For this review, take the finished solid that the model builds, in its own axes (mm). A direction names the side the tool comes from. Coordinates: 2 decimals unless noted, no trailing zeros. Loops run counter-clockwise (first coordinate to the right, second up) from the corner with the lowest first, then second, coordinate; pieces in that order, holes last. Notation, with made-up numbers: (-17, -32.5) -> (-9, -32.5) arc R23 cw to (-9, -16.5) -> close; hole circle Ø3 at (76, -13.75). An arc over 180 degrees is marked (long way). One line per item, written item: value.
from build123d import *

# Parameters (mm, degrees)
SKETCH_W      = 102.2
SKETCH_H      = 83
SKETCH_W_2    = 30
SKETCH_H_2    = 5
SKETCH_W_3    = 2
SKETCH_H_3    = 25
PAD_DEPTH     = 2
SKETCH001_R   = 2.4
SKETCH001_R_2 = 1.2
PAD001_DEPTH  = 6.2
PAD002_DEPTH  = 6.9
PAD003_DEPTH  = 1
SKETCH004_W   = 1.45
SKETCH004_H   = 11.2
PAD004_DEPTH  = 5
SKETCH005_W   = 1.45
SKETCH005_H   = 5
PAD005_DEPTH  = 5
PAD006_DEPTH  = 5
SKETCH007_W   = 107
SKETCH007_H   = 26.1
SKETCH007_W_2 = 102.2
SKETCH007_H_2 = 21.7
PAD007_DEPTH  = 5
SKETCH008_W   = 27
SKETCH008_H   = 2.75
PAD008_DEPTH  = 3.8
CHAMFER_SIZE  = 1
SKETCH009_W   = 46.5
SKETCH009_H   = 26.1
SKETCH009_W_2 = 42.1
SKETCH009_H_2 = 21.7
PAD009_DEPTH  = 5
SKETCH010_W   = 2
SKETCH010_H   = 21.75
PAD010_DEPTH  = 3.8
FILLET_R      = 1.5


with BuildPart() as part:
    # Sketch → Pad (new body)
    with BuildSketch(Plane.XY):
        Rectangle(SKETCH_W, SKETCH_H)
        with Locations((34.1, 17.5)):
            Rectangle(SKETCH_W_2, SKETCH_H_2, mode=Mode.SUBTRACT)
        with Locations((-34.1, 17.5)):
            Rectangle(SKETCH_W_2, SKETCH_H_2, mode=Mode.SUBTRACT)
        with Locations((6, -27)):
            Rectangle(SKETCH_W_3, SKETCH_H_3, mode=Mode.SUBTRACT)
        with Locations((-6, -27)):
            Rectangle(SKETCH_W_3, SKETCH_H_3, mode=Mode.SUBTRACT)
    extrude(amount=PAD_DEPTH)

    # Sketch001 (on Face22 of Pad) → Pad001 (join)
    with BuildSketch(Plane.XY.offset(2)):
        with Locations((-42.5, -25)):
            Circle(SKETCH001_R)
        with Locations((-42.5, -25)):
            Circle(SKETCH001_R_2, mode=Mode.SUBTRACT)
        with Locations((42.5, 25)):
            Circle(SKETCH001_R)
        with Locations((42.5, 25)):
            Circle(SKETCH001_R_2, mode=Mode.SUBTRACT)
    extrude(amount=PAD001_DEPTH)

    # Sketch002 → Pad002 (join)
    with BuildSketch(Plane.XY):
        Polygon((-51.1, 41.5), (51.1, 41.5), (51.1, 5.05), (53.5, 5.05), (53.5, 43.85), (-53.5, 43.85), (-53.5, 5.05), (-51.1, 5.05), align=None)
    pad002 = extrude(amount=PAD002_DEPTH)

    # Mirrored: Pad002 across XZ
    add(pad002.mirror(Plane.XZ))

    # Sketch003 (on Face36 of Mirrored) → Pad003 (join)
    with BuildSketch(Plane.XY.offset(6.9)):
        Polygon((-51.1, 5.05), (-51.1, 41.5), (51.1, 41.5), (51.1, 5.05), (52.05, 5.05), (52.05, 42.45), (-52.05, 42.45), (-52.05, 5.05), align=None)
    pad003 = extrude(amount=PAD003_DEPTH)

    # Mirrored001: Pad003 across XZ
    add(pad003.mirror(Plane.XZ))

    # Sketch004 (on Face3 of Mirrored001) → Pad004 (join)
    with BuildSketch(Plane.XY.offset(2)):
        with Locations((50.375, 0)):
            Rectangle(SKETCH004_W, SKETCH004_H)
    pad004 = extrude(amount=PAD004_DEPTH)

    # Mirrored002: Pad004 across YZ
    add(pad004.mirror(Plane.YZ))

    # Sketch005 (on Face40 of Mirrored002) → Pad005 (join)
    with BuildSketch(Plane.XY.offset(7)):
        with Locations((50.375, 0)):
            Rectangle(SKETCH005_W, SKETCH005_H)
    pad005 = extrude(amount=PAD005_DEPTH)

    # Mirrored003: Pad005 across YZ
    add(pad005.mirror(Plane.YZ))

    # Sketch006 (on Face2 of Mirrored003) → Pad006 (join)
    with BuildSketch(Plane.XZ.offset(2.5)):
        Polygon((49.65, 12), (51.1, 12), (53.1, 12), (53.1, 13), (51.15, 15.8), (49.65, 15.8), align=None)
    pad006 = extrude(amount=-PAD006_DEPTH)

    # Mirrored004: Pad006 across YZ
    add(pad006.mirror(Plane.YZ))

    # Sketch007 (on Face13 of Mirrored004) → Pad007 (join)
    with BuildSketch(Plane(origin=(0, 0, 0), x_dir=(1, 0, 0), z_dir=(0, 0, -1))):
        with Locations((0, -30.8)):
            Rectangle(SKETCH007_W, SKETCH007_H)
        with Locations((0, -30.6)):
            Rectangle(SKETCH007_W_2, SKETCH007_H_2, mode=Mode.SUBTRACT)
    extrude(amount=PAD007_DEPTH)

    # Sketch008 (on Face70 of Pad007) → Pad008 (join)
    with BuildSketch(Plane(origin=(0, 0, -5), x_dir=(1, 0, 0), z_dir=(0, 0, -1))):
        with Locations((34.1, -16.375)):
            Rectangle(SKETCH008_W, SKETCH008_H)
    pad008 = extrude(amount=-PAD008_DEPTH)

    # Mirrored005: Pad008 across YZ
    add(pad008.mirror(Plane.YZ))

    # Chamfer
    chamfer_edges = [part.edges().sort_by_distance(p)[0] for p in [
        (-34.1, 15, -1.2),
        (34.1, 15, -1.2),
    ]]
    chamfer(chamfer_edges, length=CHAMFER_SIZE)

    # Sketch009 (on Face18 of Chamfer) → Pad009 (join)
    with BuildSketch(Plane(origin=(0, 0, 0), x_dir=(1, 0, 0), z_dir=(0, 0, -1))):
        with Locations((-30.25, 30.8)):
            Rectangle(SKETCH009_W, SKETCH009_H)
        with Locations((-30.05, 30.6)):
            Rectangle(SKETCH009_W_2, SKETCH009_H_2, mode=Mode.SUBTRACT)
    pad009 = extrude(amount=PAD009_DEPTH)

    # Mirrored006: Pad009 across YZ
    add(pad009.mirror(Plane.YZ))

    # Sketch010 (on Face66 of Mirrored006) → Pad010 (join)
    with BuildSketch(Plane(origin=(0, 0, -5), x_dir=(1, 0, 0), z_dir=(0, 0, -1))):
        with Locations((6, 28.625)):
            Rectangle(SKETCH010_W, SKETCH010_H)
    pad010 = extrude(amount=-PAD010_DEPTH)

    # Mirrored007: Pad010 across YZ
    add(pad010.mirror(Plane.YZ))

    # Fillet
    fillet_edges = [part.edges().sort_by_distance(p)[0] for p in [
        (53.5, -43.85, 0.95),
        (-53.5, -43.85, 0.95),
        (53.5, 43.85, 0.95),
        (-53.5, 43.85, 0.95),
    ]]
    fillet(fillet_edges, radius=FILLET_R)


solid = part.part
1. Insertion check: pin 1 Ø1.9 at (x, y) = (-43, -25.5) entering from +Z; pin 2 Ø1.1 at (x, z) = (20, 7.5) entering from -Y; pin 3 Ø4 at (x, y) = (3, 10.5) entering from -Z; pin 4 Ø12 at (x, y) = (31.5, -16) entering from -Z. Each pin has a flat end and moves straight along its axis. Give the tip position at first contact, or say it passes through.
Return value:
pin 1: stops at z = 8.2
pin 2: stops at y = -42.45
pin 3: stops at z = 0
pin 4: stops at z = -5
2. To check wall thickness, follow probe 1 along Y at (x, z) = (-29.5, -3.5); probe 2 along X at (y, z) = (-37, 0.25); probe 3 along Y at (x, z) = (42.5, 5). State the ranges of each line that lie inside material, in increasing order. Write a range as from..to.
Return value:
probe 1: y = -43.85..-41.45, -19.75..-17.75, 15..19.75, 41.45..43.85
probe 2: x = -53.5..-7, -5..5, 7..53.5
probe 3: y = -43.85..-41.5, 22.6..23.8, 26.2..27.4, 41.5..43.85
3. Take a section at A-A, the plane z = 5.25. Give the number of separate pieces and of enclosed holes in the cut face, and give its area (3 significant figures).
Return value:
separate pieces: 3
enclosed holes: 3
area: 911 mm2
4. For faces 5 (the cylindrical face through (41.98, 22.657, 5.057)), 6 (the flat face through (52, 5.05, 4)), 7 (the flat face through (51.1, -30, -2)), 8 (the flat face through (34, 15, -4)), list the 3-axis set-ups (+Z, -Z, +X, -X, +Y, -Y) from which the entire face can be reached by the end or side of a thin tool; tool diameter is ignored.
Return value:
face 5: +Z
face 6: +Z, -Z, +X
face 7: -Z
face 8: -Z, +X, -X
5. The part is to be moulded in two halves that separate along X. For faces 1 (the flat face through (27, -42, -5)), 2 (the flat face through (-51.1, 23, 5)), 3 (the flat face through (42, 25, 2)), 4 (the flat face through (-53.5, 28, 1)), say which applies: pulls with the +X half, pulls with the -X half, needs draft (parallel to the pull), parting line crosses it, or undercut.
Return value:
face 1: needs draft
face 2: undercut
face 3: undercut
face 4: pulls with the -X half
6. Take a section at C-C, the plane y = 25. Give the boundary of the cut face in (x, z), and give its area (3 significant figures).
Return value:
outline: (-53.5, -5) -> (-51.1, -5) -> (-51.1, 0) -> (51.1, 0) -> (51.1, -5) -> (53.5, -5) -> (53.5, 6.9) -> (52.05, 6.9) -> (52.05, 7.9) -> (51.1, 7.9) -> (51.1, 2) -> (44.9, 2) -> (44.9, 8.2) -> (43.7, 8.2) -> (43.7, 2) -> (41.3, 2) -> (41.3, 8.2) -> (40.1, 8.2) -> (40.1, 2) -> (-51.1, 2) -> (-51.1, 7.9) -> (-52.05, 7.9) -> (-52.05, 6.9) -> (-53.5, 6.9) -> close
area: 278 mm2
